```python
from build123d import *

# Parameters (mm, degrees)
SKETCH1_R           = 3.175
SKETCH1_R_2         = 4.025
BOSS_EXTRUDE1_DEPTH = 6.35


with BuildPart() as part:
    # Sketch1 → Boss-Extrude1 (new body)
    with BuildSketch(Plane.XY):
        with BuildLine():
            Line((91.860390313, -8.599854689), (3.001735639, 12.7))
            Line((3.001735639, 12.7), (-48.8, 12.7))
            ThreePointArc((-48.8, 12.7), (-50.214213562, 12.114213562), (-50.8, 10.7))
            Line((-50.8, 10.7), (-50.8, -10.7))
            ThreePointArc((-50.8, -10.7), (-50.214213562, -12.114213562), (-48.8, -12.7))
            Line((-48.8, -12.7), (0, -12.7))
            Line((0, -12.7), (85.939609687, -33.300145311))
            ThreePointArc((85.939609687, -33.300145311), (101.250145311, -23.910390313), (91.860390313, -8.599854689))
        make_face()
        with Locations((-25.4, 0)):
            Circle(SKETCH1_R, mode=Mode.SUBTRACT)
        with Locations((88.9, -20.95)):
            Circle(SKETCH1_R_2, mode=Mode.SUBTRACT)
        with Locations((-44.45, 0)):
            Circle(SKETCH1_R, mode=Mode.SUBTRACT)
        with Locations((-6.35, 0)):
            Circle(SKETCH1_R, mode=Mode.SUBTRACT)
    extrude(amount=BOSS_EXTRUDE1_DEPTH)


solid = part.part
```
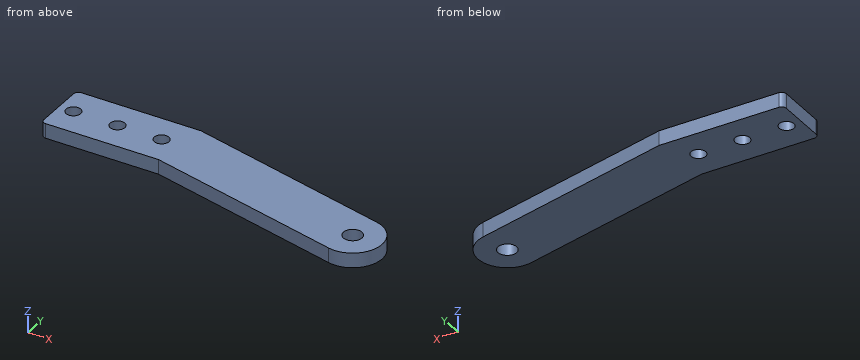
For this review, take the finished solid that the model builds, in its own axes (mm). Give positions to 0.01 mm unless a question says otherwise; leave off trailing zeros. Write each loop counter-clockwise with the first axis right and the second up, starting at its lowest first coordinate (ties: lowest second). Pieces come first, ordered by that corner, then holes. Notation, with made-up numbers: M 49.25,-37 L 63.25,-37 A23 cw 63.25,-4 Z; hole C 79.25,11.25 d8. An arc over 180 degrees is marked long. Answer as a JSON object with one key per item and string values. Group by question number.
Item 1: Consider section D-D on y = 0. Write out the cut boundary in (x, z) (3 decimals), plus the area to 3 significant figures.
Item 2: Consider section A-A on x = -44.45. Write out the cut boundary in (y, z) (3 decimals).
Item 3: Consider section C-C on y = -20.95. Write out the cut boundary in (x, z) (3 decimals).
Item 4: Consider section B-B on z = 3.75. Write out the cut boundary in (x, y) (3 decimals), plus the area to 3 significant figures.
Item 5: For pin 1 Ø1 at (x, z) = (53.5, 2.5) entering from +Y; pin 2 Ø3 at (x, z) = (23, 4) entering from -Y; pin 3 Ø1.9 at (x, z) = (-30.5, 2) entering from -Y, all flat-tipped, find the tip position at first contact; note any pin that passes through.
Item 6: For probe 1 along Y at (x, z) = (-44.45, 4.75) (3 decimals); probe 2 along Y at (x, z) = (87.5, 2); probe 3 along Y at (x, z) = (-14, 5.5), list the stretches that pass through material, from the lowest coordinate up. Write a range as [from, to].
Check result:
{
 "1": {"outline": "M -50.8,0 L -47.625,0 L -47.625,6.35 L -50.8,6.35 Z; M -41.275,0 L -28.575,0 L -28.575,6.35 L -41.275,6.35 Z; M -22.225,0 L -9.525,0 L -9.525,6.35 L -22.225,6.35 Z; M -3.175,0 L 55.984,0 L 55.984,6.35 L -3.175,6.35 Z", "area": "557 mm^2"},
 "2": {"outline": "M -12.7,0 L -3.175,0 L -3.175,6.35 L -12.7,6.35 Z; M 3.175,0 L 12.7,0 L 12.7,6.35 L 3.175,6.35 Z"},
 "3": {"outline": "M 34.417,0 L 84.875,0 L 84.875,6.35 L 34.417,6.35 Z; M 92.925,0 L 101.6,0 L 101.6,6.35 L 92.925,6.35 Z"},
 "4": {"outline": "M -50.8,-10.7 A2 ccw -48.8,-12.7 L 0,-12.7 L 85.94,-33.3 A12.7 ccw 91.86,-8.6 L 3.002,12.7 L -48.8,12.7 A2 ccw -50.8,10.7 Z; hole C -44.45,0 d6.35; hole C -25.4,0 d6.35; hole C -6.35,0 d6.35; hole C 88.9,-20.95 d8.05", "area": "3,720 mm^2"},
 "5": {"pin 1": "stops at y = 0.72", "pin 2": "stops at y = -18.57", "pin 3": "stops at y = -12.7"},
 "6": {"probe 1": "y = [-12.7, -3.175], [3.175, 12.7]", "probe 2": "y = [-33.57, -24.72], [-17.18, -7.55]", "probe 3": "y = [-12.7, 12.7]"}
}
